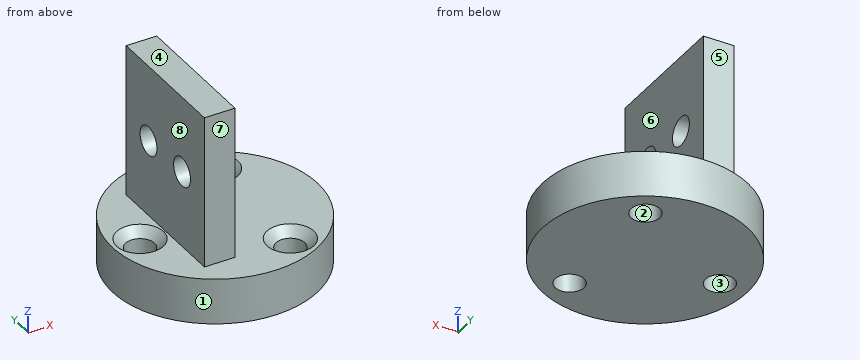
```python
from build123d import *

# Parameters (mm, degrees)
SKETCH2_R            = 8.509
BOSS_EXTRUDE1_DEPTH  = 3.81
SKETCH4_W            = 2.54
SKETCH4_H            = 11.1125
BOSS_EXTRUDE2_DEPTH  = 12.7
M2_CLEARANCE_HOLE1_D = 2.4
M2_CLEARANCE_HOLE2_D = 2.4
CHAMFER1_SIZE        = 0.75
CHAMFER2_SIZE        = 0.75
CHAMFER3_SIZE        = 0.75


with BuildPart() as part:
    # Sketch2 → Boss-Extrude1 (new body)
    with BuildSketch(Plane.XY):
        Circle(SKETCH2_R)
    extrude(amount=BOSS_EXTRUDE1_DEPTH)

    # Sketch4 → Boss-Extrude2 (add)
    with BuildSketch(Plane.XY.offset(3.81)):
        with Locations((-2.8575, 0)):
            Rectangle(SKETCH4_W, SKETCH4_H)
    extrude(amount=BOSS_EXTRUDE2_DEPTH)

    # M2 Clearance Hole1 (through all)
    with Locations(Plane.XY.offset(3.81)):
        with Locations((-6.223, 0), (3.1115, 5.389276088), (3.1115, -5.389276088)):
            Hole(M2_CLEARANCE_HOLE1_D / 2)

    # M2 Clearance Hole2 (through all)
    with Locations(Plane(origin=(-1.5875, 0, 0), x_dir=(0, 0, -1), z_dir=(1, 0, 0))):
        with Locations((-10.16, -2.38125), (-10.16, 2.38125)):
            Hole(M2_CLEARANCE_HOLE2_D / 2)

    # Chamfer1
    chamfer1_edges = [part.edges().sort_by_distance(p)[0] for p in [
        (4.3115, -5.389276088, 3.81),
    ]]
    chamfer(chamfer1_edges, length=CHAMFER1_SIZE)

    # Chamfer2
    chamfer2_edges = [part.edges().sort_by_distance(p)[0] for p in [
        (4.3115, 5.389276088, 3.81),
    ]]
    chamfer(chamfer2_edges, length=CHAMFER2_SIZE)

    # Chamfer3
    chamfer3_edges = [part.edges().sort_by_distance(p)[0] for p in [
        (-5.023, 0, 3.81),
    ]]
    chamfer(chamfer3_edges, length=CHAMFER3_SIZE)


solid = part.part
```
Input: part model. Units: mm. Frame: model coordinates. Face numbers are marked on the shaded views. A direction names the side the tool comes from. Give positions to 0.01 mm unless a question says otherwise; leave off trailing zeros. Order: outer loops, then holes, each group sorted by start corner. A loop starts at its lowest first (then second) coordinate and runs counter-clockwise, first axis right, second up.
1. Cut plane C-C (x = -3). Return loops of the section in (y, z).
Computed:
outline: (-7.96, 0) - (7.96, 0) - (7.96, 3.81) - (5.56, 3.81) - (5.56, 16.51) - (-5.56, 16.51) - (-5.56, 3.81) - (-7.96, 3.81) - close; hole circle Ø2.4 at (-2.38, 10.16); hole circle Ø2.4 at (2.38, 10.16)
2. Cut plane A-A (z = 10.16). Return loops of the section in (x, y), and give its area (3 significant figures).
Computed:
outline: (-4.13, -5.56) - (-1.59, -5.56) - (-1.59, -3.58) - (-4.13, -3.58) - close; (-4.13, -1.18) - (-1.59, -1.18) - (-1.59, 1.18) - (-4.13, 1.18) - close; (-4.13, 3.58) - (-1.59, 3.58) - (-1.59, 5.56) - (-4.13, 5.56) - close
area: 16.0 mm2
3. Set-up query: the marked faces 5, 6, 7 and 8. Return all of +Z, -Z, +X, -X, +Y, -Y with unobstructed straight access to the full face (end or side cutting, diameter ignored); none if empty.
Computed:
face 5: +Z, +X, -X, +Y
face 6: +Z, +X, +Y, -Y
face 7: +Z, +X, -X, -Y
face 8: +Z, -X, +Y, -Y
4. Line query: probe 1 along Y at (x, z) = (-2.2, 10.16); probe 2 along Z at (x, y) = (1.75, -3.5); probe 3 along X at (y, z) = (0, 5.25). Output: solid intervals per line, ascending.
Computed:
probe 1: y = -5.56 to -3.58, -1.18 to 1.18, 3.58 to 5.56
probe 2: z = 0 to 3.81
probe 3: x = -4.13 to -1.59
5. Cut plane B-B (y = 0). Return loops of the section in (x, z).
Computed:
outline: (-8.51, 0) - (-7.42, 0) - (-7.42, 3.06) - (-8.17, 3.81) - (-8.51, 3.81) - close; (-5.02, 0) - (8.51, 0) - (8.51, 3.81) - (-1.59, 3.81) - (-1.59, 16.51) - (-4.13, 16.51) - (-4.13, 3.81) - (-4.27, 3.81) - (-5.02, 3.06) - close
6. Pin query (flat end, axial travel): pin 1 Ø5.5 at (y, z) = (2, 9) entering from +X; pin 2 Ø3 at (x, y) = (3.11, 5.39) entering from +Z; pin 3 Ø4 at (x, y) = (-6.223, 0) entering from +Z. Return the tip coordinate at first contact, or that it passes through.
Computed:
pin 1: stops at x = -1.59
pin 2: stops at z = 3.36
pin 3: stops at z = 3.81
7. Cut plane D-D (y = 2.75). Return loops of the section in (x, z), and give its area (3 significant figures).
Computed:
outline: (-8.05, 0) - (8.05, 0) - (8.05, 3.81) - (-1.59, 3.81) - (-1.59, 9.02) - (-4.13, 9.02) - (-4.13, 3.81) - (-8.05, 3.81) - close; (-4.13, 11.3) - (-1.59, 11.3) - (-1.59, 16.51) - (-4.13, 16.51) - close
area: 87.8 mm2
8. Draft query along X for the marked faces 1, 2, 3 and 4. Return one class per face: released by +X, released by -X, zero draft, split by the parting line, or undercut.
Computed:
face 1: split by the parting line
face 2: undercut
face 3: undercut
face 4: zero draft
